Autodesk Inventor part; units mm, degrees
ref_plane "YZ Plane" through (0, 0, 0) normal (1, 0, 0) x (0, 1, 0)
ref_plane "XZ Plane" through (0, 0, 0) normal (0, 1, 0) x (-1, 0, 0)
ref_plane "XY Plane" through (0, 0, 0) normal (0, 0, 1) x (1, 0, 0)
sketch "Sketch2" plane through (0, 0, 0) normal (0, 1, 0) x (-1, 0, 0)
  arc A0 (44.45, 506.057) -> (-44.45, 506.057) centre (0, -1.4242) ccw construction
  arc A1 (44.45, 506.057) -> (-44.45, 506.057) centre (0, -1.4242) ccw
  line L0 (44.45, 84.2423) -> (44.45, 506.057)
  line L1 (-44.45, 506.057) -> (-44.45, 84.2423)
  circle A2 centre (0, 0) radius 57.15 construction
  circle A3 centre (0, 0) radius 63.5
  arc A4 (-44.45, 84.2423) -> (44.45, 84.2423) centre (0, 0) ccw
  line L2 (0, 0) -> (0, 508) construction
  arc A5 (31.75, 494.2843) -> (-31.75, 494.2843) centre (0, -1.4242) ccw
  line L3 (-31.75, 494.2843) -> (-31.75, 69.85)
  arc A6 (-31.75, 77.0401) -> (31.75, 77.0401) centre (0, 0) ccw construction
  line L4 (31.75, 69.85) -> (31.75, 494.2843)
  arc A7 (31.75, 62.217) -> (-31.75, 62.217) centre (0, 0) ccw construction
  line L5 (0, 69.85) -> (0, 63.5) construction
  line L6 (-31.75, 69.85) -> (31.75, 69.85)
  point P0 (-7.0927, 251.5509)
  dimension "d23" = 127
  dimension "d21" = 88.9
  dimension "d22" = 114.3
  dimension "d24" = 190.5
  dimension "d25" = 508
  dimension "d26" = 88.9
  dimension "d29" = 12.7
  dimension "d31" = 139.7
  dimension "d69" = 12.7
  dimension "d70" = 12.7
extrude "Extrusion2" add sketch "Sketch2" along normal blind 12.7
sketch "Sketch3" plane through (0, 12.7, 0) normal (0, 1, 0) x (1, 0, 0)
  arc A0 (-44.4483, -506.0602) -> (44.4517, -506.0602) centre (0.0017, 1.4211) ccw construction
  line L0 (44.4517, -506.0602) -> (44.4517, -84.2454) construction
  line L1 (-44.4483, -506.0602) -> (44.4517, -506.0602) construction
  line L2 (44.4517, -506.0602) -> (44.4517, -84.2454) construction
  line L3 (44.4517, -84.2454) -> (-44.4483, -84.2454) construction
  line L4 (-44.4483, -84.2454) -> (-44.4483, -506.0602) construction
  line L5 (-44.4483, -84.2454) -> (-44.4483, -506.0602) construction
  line L6 (-44.4483, -295.1528) -> (-38.0983, -295.1528) construction
  line L7 (-38.0983, -295.1528) -> (-38.0983, -506.0602) construction
  line L8 (-38.0983, -295.1528) -> (-38.0983, -84.2454) construction
  circle A1 centre (-38.0983, -96.9454) radius 3.175
  circle A2 centre (-38.0983, -480.6602) radius 3.175
  circle A3 centre (-38.0983, -295.1528) radius 3.175
  line L9 (0.0017, -506.0602) -> (0.0017, 1.4211) construction
  circle A4 centre (38.1017, -295.1528) radius 3.175
  line L10 (44.4517, -295.1528) -> (38.1017, -295.1528) construction
  circle A5 centre (38.1017, -96.9454) radius 3.175
  circle A6 centre (38.1017, -480.6602) radius 3.175
  line L11 (38.1017, -295.1528) -> (38.1017, -506.0602) construction
  line L12 (38.1017, -295.1528) -> (38.1017, -84.2454) construction
  line L13 (44.4517, -84.2454) -> (44.4517, -506.0602) construction
  line L14 (44.4517, -84.2454) -> (44.4517, -506.0602) construction
  point P0 (0, 0)
  dimension "d54" = 6.35
  dimension "d55" = 90
  dimension "d56" = 6.35
  dimension "d57" = 12.7
  dimension "d58" = 6.35
  dimension "d59" = 6.35
  dimension "d60" = 25.4
extrude "Extrusion3" cut sketch "Sketch3" against normal blind 12.7
equation "\"d26\" = d21"
properties part number "Arm Layer 3"
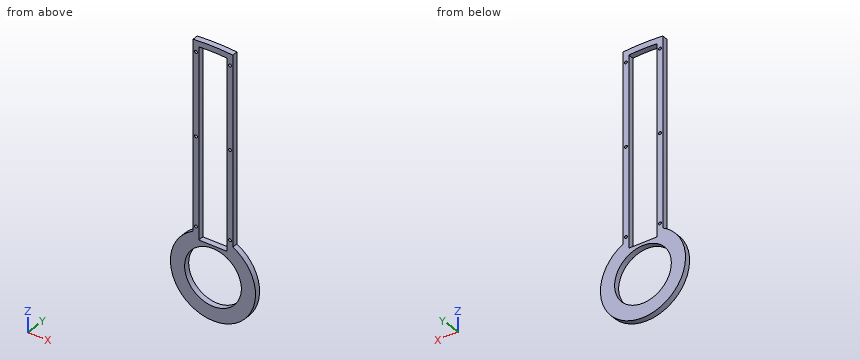
Geometry check sheet. Reference: the model listing, model coordinates, mm. Coordinates: 2 decimals unless noted, no trailing zeros. Write each loop counter-clockwise with the first axis right and the second up, starting at its lowest first coordinate (ties: lowest second). Pieces come first, ordered by that corner, then holes. Notation, with made-up numbers: M 67.5,-27.5 L 112.5,-27.5 A28 ccw 112.5,5.5 Z; hole C 16,-39 d10. An arc over 180 degrees is marked long. One line per item, written item: value. Start each with the question number.
(1) Sectioned sample at C-C, the plane y = 7. State how many separate pieces and enclosed holes the cut face has, and give its area (3 significant figures).
(2) Depth check by flat-ended pin: pin 1 (4 mm diameter, centred on y = 8.5, z = 103, fed in from -X); pin 2 (6.5 mm diameter, centred on y = 4, z = 176.5, fed in from +X); pin 3 (4 mm diameter, centred on x = 38.1, z = 480.66, fed in from -Y); pin 4 (5 mm diameter, centred on y = 3.5, z = 72.5, fed in from +X). Enter the tip coordinate at first touch or a pass-through.
(3) Sectioned sample at A-A, the plane z = 0. Enter the section's corners in (x, y), and give its area (3 significant figures).
(4) Sectioned sample at B-B, the plane x = -20.5. Enter the section's corners in (y, z), and give its area (3 significant figures).
(5) Scan lines: line 1 along Z through (x, y) = (-1, 9.5); line 2 along X through (y, z) = (1.5, 213.5); line 3 along Z through (x, y) = (13, 9). Record each from-to range of solid material in increasing order. Write a range as [from, to].
(6) Sectioned sample at D-D, the plane x = -58. Enter the section's corners in (y, z), and give its area (3 significant figures).
Filled sheet:
1. separate pieces: 1
1. enclosed holes: 8
1. area: 25,600 mm²
2. pin 1: x = -44.45
2. pin 2: x = 44.45
2. pin 3: through
2. pin 4: x = 64.6
3. outline: M -95.25,0 L -63.5,0 L -63.5,12.7 L -95.25,12.7 Z; M 63.5,0 L 95.25,0 L 95.25,12.7 L 63.5,12.7 Z
3. area: 806 mm²
4. outline: M 0,-93.02 L 12.7,-93.02 L 12.7,-60.1 L 0,-60.1 Z; M 0,60.1 L 12.7,60.1 L 12.7,69.85 L 0,69.85 Z; M 0,494.88 L 12.7,494.88 L 12.7,507.59 L 0,507.59 Z
4. area: 703 mm²
5. line 1: [-95.24, -63.49], [63.49, 69.85], [495.3, 508]
5. line 2: [-44.45, -31.75], [31.75, 44.45]
5. line 3: [-94.36, -62.16], [62.16, 69.85], [495.13, 507.83]
6. outline: M 0,-75.56 L 12.7,-75.56 L 12.7,-25.85 L 0,-25.85 Z; M 0,25.85 L 12.7,25.85 L 12.7,75.56 L 0,75.56 Z
6. area: 1,260 mm²
